from build123d import *

# Parameters (mm, degrees)
SKETCH_1_W                  = 30
SKETCH_1_H                  = 11
EXTRUDE_1_DEPTH             = 6
SKETCH_2_W                  = 16
SKETCH_2_H                  = 2
CUT_EXTRUDE_1_DEPTH         = 144
EXTRUDE_2_DEPTH             = 80
SKETCH_4_R                  = 1.75
CUT_EXTRUDE_2_DEPTH         = 144
SKETCH_5_W                  = 11
SKETCH_5_H                  = 86
CUT_EXTRUDE_3_DEPTH         = 2.5
EXTRUDE_3_REACH             = 83.58
EXTRUDE_3_DIRECTION_2_REACH = 83.58
SKETCH_7_W                  = 1.5
SKETCH_7_H                  = 86
EXTRUDE_4_DEPTH             = 10
CUT_EXTRUDE_4_DEPTH         = 40
EXTRUDE_5_DEPTH             = 2
SKETCH_10_R                 = 1.25
CUT_EXTRUDE_5_DEPTH         = 3
SKETCH_11_W                 = 3
SKETCH_11_H                 = 86
EXTRUDE_6_DEPTH             = 12.5
SKETCH_12_W                 = 10
SKETCH_12_H                 = 2
EXTRUDE_7_DEPTH             = 12.5
SKETCH_13_R                 = 1.65
CUT_EXTRUDE_6_DEPTH         = 100


with BuildPart() as part:
    # 草图1 → 凸台-拉伸1 (new body)
    with BuildSketch(Plane(origin=(0, 0, 0), x_dir=(1, 0, 0), z_dir=(0, 1, 0))):
        Rectangle(SKETCH_1_W, SKETCH_1_H)
    extrude(amount=EXTRUDE_1_DEPTH)

    # 草图2 → 切除-拉伸1 (cut)
    with BuildSketch(Plane.ZY.offset(15)):
        with Locations((-5.5, 3)):
            Rectangle(SKETCH_2_W, SKETCH_2_H)
    extrude(amount=-CUT_EXTRUDE_1_DEPTH, mode=Mode.SUBTRACT)

    # 草图3 → 凸台-拉伸2 (add)
    with BuildSketch(Plane(origin=(0, 6, 0), x_dir=(1, 0, 0), z_dir=(0, 1, 0))):
        Polygon((2, 5.5), (-2, 5.5), (-2, -3.5), (-15, -3.5), (-15, -5.5), (15, -5.5), (15, -3.5), (2, -3.5), align=None)
    extrude(amount=EXTRUDE_2_DEPTH)

    # 草图4 → 切除-拉伸2 (cut)
    with BuildSketch(Plane(origin=(0, 6, 0), x_dir=(1, 0, 0), z_dir=(0, 1, 0))):
        with Locations(Location((-7.5, 2, 0), (0, 0, 270))):
            Circle(SKETCH_4_R)
        with Locations(Location((7.5, 2, 0), (0, 0, 270))):
            Circle(SKETCH_4_R)
    extrude(amount=-CUT_EXTRUDE_2_DEPTH, mode=Mode.SUBTRACT)

    # 草图5 → 切除-拉伸3 (cut)
    with BuildSketch(Plane.ZY.offset(15)):
        with Locations((0, 43)):
            Rectangle(SKETCH_5_W, SKETCH_5_H)
    extrude(amount=-CUT_EXTRUDE_3_DEPTH, mode=Mode.SUBTRACT)

    # 凸台-拉伸3: up to this face of the body (flat: up to its plane)
    extrude_3_end = Plane(part.part.faces().sort_by_distance((0.755494505, 86, 2.324175824))[0])
    # 草图6 → 凸台-拉伸3 (add, up to the picked face)
    with BuildSketch(Plane(origin=(0, 6, 0), x_dir=(1, 0, 0), z_dir=(0, 1, 0)), mode=Mode.PRIVATE) as extrude_3_sk1:
        with BuildLine():
            Line((-22.5, 7.5), (-25.5, 7.5))
            ThreePointArc((-25.5, 7.5), (-21.692388155, -1.692388155), (-12.5, -5.5))
            Line((-12.5, -5.5), (-12.5, -2.5))
            ThreePointArc((-12.5, -2.5), (-19.571067812, 0.428932188), (-22.5, 7.5))
        make_face()
    extrude_3_tool1 = split(extrude(extrude_3_sk1.sketch, amount=EXTRUDE_3_REACH, mode=Mode.PRIVATE), bisect_by=extrude_3_end, keep=Keep.BOTH, mode=Mode.PRIVATE)
    add(extrude_3_tool1.solids().sort_by(Axis((-19.862646, 6, -0.137354), (0, 1, 0)))[0])

    # 凸台-拉伸3 direction 2: up to this face of the body (flat: up to its plane)
    extrude_3_direction_2_end = Plane(part.part.faces().sort_by_distance((1.334914955, 0, 0.135863928))[0])
    # 草图6 → 凸台-拉伸3 direction 2 (add, up to the picked face)
    with BuildSketch(Plane(origin=(0, 6, 0), x_dir=(1, 0, 0), z_dir=(0, 1, 0)), mode=Mode.PRIVATE) as extrude_3_direction_2_sk1:
        with BuildLine():
            Line((-22.5, 7.5), (-25.5, 7.5))
            ThreePointArc((-25.5, 7.5), (-21.692388155, -1.692388155), (-12.5, -5.5))
            Line((-12.5, -5.5), (-12.5, -2.5))
            ThreePointArc((-12.5, -2.5), (-19.571067812, 0.428932188), (-22.5, 7.5))
        make_face()
    extrude_3_direction_2_tool1 = split(extrude(extrude_3_direction_2_sk1.sketch, amount=-EXTRUDE_3_DIRECTION_2_REACH, mode=Mode.PRIVATE), bisect_by=extrude_3_direction_2_end, keep=Keep.BOTH, mode=Mode.PRIVATE)
    add(extrude_3_direction_2_tool1.solids().sort_by(Axis((-19.862646, 6, -0.137354), (0, -1, 0)))[0])

    # 草图7 → 凸台-拉伸4 (add)
    with BuildSketch(Plane(origin=(0, 0, -7.5), x_dir=(-1, 0, 0), z_dir=(0, 0, -1))):
        with Locations((23.25, 43)):
            Rectangle(SKETCH_7_W, SKETCH_7_H)
    extrude(amount=EXTRUDE_4_DEPTH)

    # 草图8 → 切除-拉伸4 (cut)
    with BuildSketch(Plane(origin=(-12.5, 0, 0), x_dir=(0, 0, -1), z_dir=(1, 0, 0))):
        Polygon((26.892505746, 86), (-2.5, 86), (-2.5, 6), (-2.5, -9.514717226), (26.892505746, -9.514717226), align=None)
        Polygon((-3.5, 6), (-3.5, 86), (-26.700940199, 86), (-26.700940199, -9.514717226), (-2.5, -9.514717226), (-2.5, 6), align=None)
    extrude(amount=CUT_EXTRUDE_4_DEPTH, mode=Mode.SUBTRACT)


with BuildPart() as cut_extrude_4_kept_piece:
    # of the separate pieces the step leaves, the one the design keeps (cut_extrude_4_pieces_kept)
    add(part.part.solids().sort_by_distance((-22.5, 0, -7.5))[0])

    # 草图9 → 凸台-拉伸5 (add)
    with BuildSketch(Plane(origin=(0, 86, 0), x_dir=(1, 0, 0), z_dir=(0, 1, 0))):
        with BuildLine():
            Line((-12.5, -2.5), (-12.5, 7.5))
            Line((-12.5, 7.5), (-22.5, 7.5))
            ThreePointArc((-22.5, 7.5), (-19.571067812, 0.428932188), (-12.5, -2.5))
        make_face()
    extrude_5 = extrude(amount=-EXTRUDE_5_DEPTH)

    # 草图10 → 切除-拉伸5 (cut)
    with BuildSketch(Plane(origin=(0, 84, 0), x_dir=(-1, 0, 0), z_dir=(0, -1, 0))):
        with Locations(Location((14.8, 2.5, 0), (0, 0, 90))):
            Circle(SKETCH_10_R)
        with Locations(Location((17.5, 5.2, 0), (0, 0, 90))):
            Circle(SKETCH_10_R)
    cut_extrude_5 = extrude(amount=-CUT_EXTRUDE_5_DEPTH, mode=Mode.SUBTRACT)

    # 镜向2: 凸台-拉伸5, 切除-拉伸5 across plane
    add(extrude_5.mirror(Plane(origin=(0, 43, 0), x_dir=(0, 0, 1), z_dir=(0, -1, 0))))
    add(cut_extrude_5.mirror(Plane(origin=(0, 43, 0), x_dir=(0, 0, 1), z_dir=(0, -1, 0))), mode=Mode.SUBTRACT)

    # 草图11 → 凸台-拉伸6 (add)
    with BuildSketch(Plane(origin=(-12.5, 0, 0), x_dir=(0, 0, -1), z_dir=(1, 0, 0))):
        with Locations((-4, 43)):
            Rectangle(SKETCH_11_W, SKETCH_11_H)
    extrude(amount=EXTRUDE_6_DEPTH)

    # 草图12 → 凸台-拉伸7 (add)
    with BuildSketch(Plane(origin=(-12.5, 0, 0), x_dir=(0, 0, -1), z_dir=(1, 0, 0))):
        with Locations((2.5, 1)):
            Rectangle(SKETCH_12_W, SKETCH_12_H)
        with Locations((2.5, 85)):
            Rectangle(SKETCH_12_W, SKETCH_12_H)
    extrude(amount=EXTRUDE_7_DEPTH)

    # 草图13 → 切除-拉伸6 (cut)
    with BuildSketch(Plane(origin=(0, 86, 0), x_dir=(1, 0, 0), z_dir=(0, 1, 0))):
        with Locations(Location((-7.5, 2, 0), (0, 0, 270))):
            Circle(SKETCH_13_R)
    extrude(amount=-CUT_EXTRUDE_6_DEPTH, mode=Mode.SUBTRACT)


solid = cut_extrude_4_kept_piece.part
Build history of the part. All positions in model axes, mm. A direction names the side the tool comes from. Round coordinates to 2 decimals unless told otherwise and drop trailing zeros. Loops run counter-clockwise (first coordinate to the right, second up) from the corner with the lowest first, then second, coordinate; pieces in that order, holes last. Notation, with made-up numbers: (31.25, 18) -> (77.25, 18) arc R23 ccw to (77.25, 54) -> close; hole circle Ø4 at (51, 66.25). An arc over 180 degrees is marked (long way). Answer in a Markdown table with one row per item.
Item 1: Pin check, flat tips, straight feed: pin 1 (1 mm diameter, centred on x = -17.5, y = 24.5, fed in from -Z); pin 2 (5 mm diameter, centred on y = 33, z = -12.5, fed in from -X); pin 3 (3 mm diameter, centred on y = 47, z = -11, fed in from +X); pin 4 (1.5 mm diameter, centred on x = -7, z = -2.5, fed in from -Y). Stop position of each tip, or through.
Answers below:
| item | result |
|---|---|
| pin 1 | stops at z = 0.85 |
| pin 2 | stops at x = -24 |
| pin 3 | stops at x = -22.5 |
| pin 4 | passes through |
Item 2: Saw through at B-B (y = 63.5). Write the cut outline in (x, z), and give its area (3 significant figures).
Answers below:
| item | result |
|---|---|
| outline | (-25.5, -7.5) -> (-24, -7.5) -> (-24, -17.5) -> (-22.5, -17.5) -> (-22.5, -7.5) arc R10 cw to (-12.5, 2.5) -> (0, 2.5) -> (0, 5.5) -> (-12.5, 5.5) arc R13 ccw to start |
| area | 107 mm² |
Item 3: Mould opens along X. For faces 5 (the cylindrical face through (-16.446, 84.986, -5.872)), 6 (the flat face through (-24, 42, -12)), 7 (the cylindrical face through (-8.964, 85.014, -1.239)), 8 (the flat face through (-11, 1, -7.5)) say: +X half, -X half, draft (parallel to the pull), parting line (faces both ways), or undercut.
Answers below:
| item | result |
|---|---|
| face 5 | undercut |
| face 6 | -X half |
| face 7 | undercut |
| face 8 | draft |
Item 4: Which spindle directions (+Z, -Z, +X, -X, +Y, -Y) get a long thin tool onto all of the face, cutting with end or side? Do faces 1 (the flat face through (-23, 44, -17.5)), 2 (the flat face through (-11, 85, -7.5)), 3 (the flat face through (-25, 44, -7.5)), 4 (the flat face through (-11, 2, -2)). Say none if no direction does.
Answers below:
| item | result |
|---|---|
| face 1 | -Z, +X, -X, +Y, -Y |
| face 2 | -Z, +X, +Y, -Y |
| face 3 | -Z, -X, +Y, -Y |
| face 4 | -Z, +X |
Item 5: Saw through at C-C (z = -5.2). Write the cut outline in (x, y), and give its area (3 significant figures).
Answers below:
| item | result |
|---|---|
| outline | (-25.29, 0) -> (-18.75, 0) -> (-18.75, 2) -> (-22.23, 2) -> (-22.23, 84) -> (-18.75, 84) -> (-18.75, 86) -> (-25.29, 86) -> close; (-16.25, 0) -> (0, 0) -> (0, 2) -> (-16.25, 2) -> close; (-16.25, 84) -> (0, 84) -> (0, 86) -> (-16.25, 86) -> close |
| area | 342 mm² |
Item 6: Saw through at D-D (x = -11.75). Write the cut outline in (y, z), and give its area (3 significant figures).
Answers below:
| item | result |
|---|---|
| outline | (0, -7.5) -> (2, -7.5) -> (2, 2.5) -> (84, 2.5) -> (84, -7.5) -> (86, -7.5) -> (86, 5.5) -> (0, 5.5) -> close |
| area | 298 mm² |
Item 7: Drill centre lines: L1, parallel to X at y = 1.6, z = -2.5; L2, parallel to Y at x = -19, z = -5.75; L3, parallel to Z at x = -11, y = 29. Where is each one in solid material? Low to high. Write a range as [from, to].
Answers below:
| item | result |
|---|---|
| L1 | x = [-24.5, -16.05], [-13.55, -9.07], [-5.93, 0] |
| L2 | y = [0, 2], [84, 86] |
| L3 | z = [2.5, 5.5] |
Item 8: Saw through at A-A (x = -17.5). Write the cut outline in (y, z).
Answers below:
| item | result |
|---|---|
| outline | (0, -7.5) -> (2, -7.5) -> (2, -6.45) -> (0, -6.45) -> close; (0, -3.95) -> (2, -3.95) -> (2, 1.16) -> (84, 1.16) -> (84, -3.95) -> (86, -3.95) -> (86, 4.5) -> (0, 4.5) -> close; (84, -7.5) -> (86, -7.5) -> (86, -6.45) -> (84, -6.45) -> close |
